Part model, mm, in its own coordinate system. A direction names the side the tool comes from. Coordinates: 2 decimals unless noted, no trailing zeros. Loops run counter-clockwise (first coordinate to the right, second up) from the corner with the lowest first, then second, coordinate; pieces in that order, holes last. Notation, with made-up numbers: M 45.25,13.5 L 78.25,13.5 A18 cw 78.25,23.5 Z; hole C 48,49.25 d7. An arc over 180 degrees is marked long. Use a Markdown table: item, result. Add a question column.
1) Band-saw the part on D-D (z = 101.6). List the corners of the cut face in (x, y) (3 decimals), plus the area to 3 significant figures.
2) Band-saw the part on C-C (z = -101.6). List the corners of the cut face in (x, y) (3 decimals), plus the area to 3 significant figures.
3) Wall check: probe 1 along X at (y, z) = (16, -24) (3 decimals); probe 2 along Y at (x, z) = (-131, 0) (3 decimals); probe 3 along X at (y, z) = (1.65, -101.6) (3 decimals). Give the ranges that are in metal, low to high. Write a range as from..to.
4) Band-saw the part on A-A (x = 0). List the corners of the cut face in (y, z) (3 decimals).
5) Tool access for faces 1 (the cylindrical face through (-2.2, 1.61, 111.52)), 2 (the flat face through (79.375, 18, 1)): list every direction of +Z, -Z, +X, -X, +Y, -Y with a clear straight run to the whole face (end or side of a thin tool).
6) Pin check, flat tips, straight feed: pin 1 Ø3 at (x, y) = (83.5, 27) entering from +Z; pin 2 Ø4 at (y, z) = (26.5, -23) entering from -X (3 decimals); pin 3 Ø2.5 at (x, y) = (108, 2) entering from +Z. Stop position of each tip, or through.
7) Pull direction X, two halves, no side cores. Call faces 3 (the flat face through (136.525, 18, 1)), 4 (the flat face through (85.725, 26, 1)), 5 (the flat face through (-79.375, 18, 1)), 6 (the flat face through (-136.525, 18, 1)): released by +X, released by -X, zero draft, split by the parting line, or undercut.
8) Band-saw the part on B-B (y = 14.5). List the corners of the cut face in (x, z) (3 decimals).
from build123d import *

# Parameters (mm, degrees)
SKETCH1_R           = 152.4
BOSS_EXTRUDE1_DEPTH = 3.175
SKETCH2_W           = 44.45
SKETCH2_H           = 88.9
CUT_EXTRUDE1_DEPTH  = 4.175
SKETCH3_W           = 6.35
SKETCH3_H           = 88.9
BOSS_EXTRUDE2_DEPTH = 38.1
SKETCH4_R           = 2.38125
CUT_EXTRUDE2_DEPTH  = 289.925
SKETCH5_R           = 10.16
CUT_EXTRUDE3_DEPTH  = 4.175


with BuildPart() as part:
    # Sketch1 → Boss-Extrude1 (new body)
    with BuildSketch(Plane(origin=(0, 0, 0), x_dir=(1, 0, 0), z_dir=(0, 1, 0))):
        Circle(SKETCH1_R)
    extrude(amount=BOSS_EXTRUDE1_DEPTH)

    # Sketch2 → Cut-Extrude1 (cut, through all)
    with BuildSketch(Plane(origin=(0, 3.175, 0), x_dir=(1, 0, 0), z_dir=(0, 1, 0))):
        with Locations((-107.95, 0)):
            Rectangle(SKETCH2_W, SKETCH2_H)
    cut_extrude1 = extrude(amount=-CUT_EXTRUDE1_DEPTH, mode=Mode.SUBTRACT)

    # Sketch3 → Boss-Extrude2 (add)
    with BuildSketch(Plane(origin=(0, 3.175, 0), x_dir=(1, 0, 0), z_dir=(0, 1, 0))):
        with Locations((-133.35, 0)):
            Rectangle(SKETCH3_W, SKETCH3_H)
        with Locations((-82.55, 0)):
            Rectangle(SKETCH3_W, SKETCH3_H)
    boss_extrude2 = extrude(amount=BOSS_EXTRUDE2_DEPTH)

    # Mirror1: Cut-Extrude1, Boss-Extrude2 across plane
    add(cut_extrude1.mirror(Plane(origin=(0, 0, 0), x_dir=(0, 0, 1), z_dir=(1, 0, 0))), mode=Mode.SUBTRACT)
    add(boss_extrude2.mirror(Plane(origin=(0, 0, 0), x_dir=(0, 0, 1), z_dir=(1, 0, 0))))

    # Sketch4 → Cut-Extrude2 (cut, through all)
    with BuildSketch(Plane(origin=(136.525, 0, 0), x_dir=(0, 0, -1), z_dir=(1, 0, 0))):
        with Locations((0, 20.6375)):
            Circle(SKETCH4_R)
    extrude(amount=-CUT_EXTRUDE2_DEPTH, mode=Mode.SUBTRACT)

    # Sketch5 → Cut-Extrude3 (cut, through all)
    with BuildSketch(Plane(origin=(0, 3.175, 0), x_dir=(1, 0, 0), z_dir=(0, 1, 0))):
        with Locations((0, -101.6)):
            Circle(SKETCH5_R)
        with Locations((-53.975, 101.6)):
            Circle(SKETCH5_R)
        with Locations((53.975, 101.6)):
            Circle(SKETCH5_R)
    extrude(amount=-CUT_EXTRUDE3_DEPTH, mode=Mode.SUBTRACT)


solid = part.part
Entries:
| question | item | result |
|---|---|---|
| 1 | outline | M -113.592,0 L -10.16,0 L -10.16,3.175 L -113.592,3.175 Z; M 10.16,0 L 113.592,0 L 113.592,3.175 L 10.16,3.175 Z |
| 1 | area | 657 mm2 |
| 2 | outline | M -113.592,0 L -64.135,0 L -64.135,3.175 L -113.592,3.175 Z; M -43.815,0 L 43.815,0 L 43.815,3.175 L -43.815,3.175 Z; M 64.135,0 L 113.592,0 L 113.592,3.175 L 64.135,3.175 Z |
| 2 | area | 592 mm2 |
| 3 | probe 1 | -136.525..-130.175, -85.725..-79.375, 79.375..85.725, 130.175..136.525 |
| 3 | probe 2 | 0..18.256, 23.019..41.275 |
| 3 | probe 3 | -113.592..-64.135, -43.815..43.815, 64.135..113.592 |
| 4 | outline | M 0,-152.4 L 3.175,-152.4 L 3.175,91.44 L 0,91.44 Z; M 0,111.76 L 3.175,111.76 L 3.175,152.4 L 0,152.4 Z |
| 5 | face 1 | +Y, -Y |
| 5 | face 2 | +Z, -Z, +Y |
| 6 | pin 1 | z = 44.45 |
| 6 | pin 2 | x = -136.525 |
| 6 | pin 3 | z = 108.77 |
| 7 | face 3 | released by +X |
| 7 | face 4 | undercut |
| 7 | face 5 | undercut |
| 7 | face 6 | released by -X |
| 8 | outline | M -136.525,-44.45 L -130.175,-44.45 L -130.175,44.45 L -136.525,44.45 Z; M -85.725,-44.45 L -79.375,-44.45 L -79.375,44.45 L -85.725,44.45 Z; M 79.375,-44.45 L 85.725,-44.45 L 85.725,44.45 L 79.375,44.45 Z; M 130.175,-44.45 L 136.525,-44.45 L 136.525,44.45 L 130.175,44.45 Z |
